Check sheet for the modelled part. Datum: model origin and axes. Units: mm. Face numbers are marked on the shaded views. A direction names the side the tool comes from. Round coordinates to 2 decimals unless told otherwise and drop trailing zeros.
Q1. Depth check by flat-ended pin: P1, Ø2, axis at x = 16, y = 59, coming from the +Z side; P2, Ø4, axis at x = 54.5, z = 3.5, coming from the -Y side; P3, Ø1.5, axis at x = 19.5, z = 23, coming from the -Y side. Enter the tip coordinate at first touch or a pass-through.
Q2. Set-up check for the marked faces 1 and 2: record each of +Z, -Z, +X, -X, +Y, -Y from which the full face is reachable in a straight line by a thin tool's end or side.
Q3. Scan lines: probe 1 along Y at (x, z) = (70.5, 4); probe 2 along Z at (x, y) = (26.5, 29); probe 3 along Z at (x, y) = (8.5, 72.5). Record each from-to range of solid material in increasing order.
Q4. Cross-section at A-A on x = 72.5. Give the number of separate pieces and of enclosed holes in the cut face, then the cut area to 3 significant figures.
Autodesk Fusion 360 part; units mm, degrees
sketch "Sketch1" plane through (0, 0, 0) normal (1, 0, 0) x (0, 1, 0)
  line L0 (0, 0) -> (90, 0)
  line L1 (0, 0) -> (77.7817, 77.7817)
  line L2 (77.7817, 77.7817) -> (81.3173, 74.2462)
  line L3 (81.3173, 74.2462) -> (12.0711, 5)
  line L4 (12.0711, 5) -> (90, 5)
  line L5 (90, 5) -> (90, 0)
  dimension "d1" = 110
  dimension "d2" = 5
  dimension "d3" = 5
  dimension "d4" = 45
  dimension "d5" = 90
extrude "Extrude1" add sketch "Sketch1" along normal blind 85
sketch "Sketch2" plane through (0, 0, 0) normal (0, -0.7071, 0.7071) x (1, 0, 0)
  line L0 (0, 110) -> (0, 0)
  line L1 (0, 0) -> (85, 0)
  line L2 (85, 0) -> (85, 110)
  line L3 (85, 110) -> (0, 110)
  line L4 (0, 12.0711) -> (85, 12.0711)
  line L5 (0, 0) -> (85, 0)
  line L6 (0, 17.0711) -> (85, 17.0711)
  line L7 (42.5, 17.0711) -> (42.5, 110) construction
  line L8 (42.5, 63.5355) -> (0, 63.5355) construction
  line L9 (15, 90) -> (70, 90)
  arc A0 (70, 90) -> (70, 100) centre (70, 95) ccw
  line L10 (70, 100) -> (15, 100)
  arc A1 (15, 100) -> (15, 90) centre (15, 95) ccw
  line L11 (15, 95) -> (70, 95) construction
  line L12 (70, 83.75) -> (15, 83.75)
  arc A2 (15, 83.75) -> (15, 73.75) centre (15, 78.75) ccw
  line L13 (15, 73.75) -> (70, 73.75)
  arc A3 (70, 73.75) -> (70, 83.75) centre (70, 78.75) ccw
  line L14 (70, 67.5) -> (15, 67.5)
  arc A4 (15, 67.5) -> (15, 57.5) centre (15, 62.5) ccw
  line L15 (15, 57.5) -> (70, 57.5)
  arc A5 (70, 57.5) -> (70, 67.5) centre (70, 62.5) ccw
  line L16 (70, 51.25) -> (15, 51.25)
  arc A6 (15, 51.25) -> (15, 41.25) centre (15, 46.25) ccw
  line L17 (15, 41.25) -> (70, 41.25)
  arc A7 (70, 41.25) -> (70, 51.25) centre (70, 46.25) ccw
  line L18 (70, 35) -> (15, 35)
  arc A8 (15, 35) -> (15, 25) centre (15, 30) ccw
  line L19 (15, 25) -> (70, 25)
  arc A9 (70, 25) -> (70, 35) centre (70, 30) ccw
  dimension "d8" = 5
  dimension "d51" = 10
  dimension "d52" = 10
  dimension "d53" = 10
  dimension "d54" = 5
  dimension "d57" = 0
  dimension "d58" = -65
extrude "Extrude2" add sketch "Sketch2" along normal blind 15 contours L0 L2 L4 L6
fillet "Fillet1" radius 2.5 1 edges at (42.5, 0, 0)
fillet "Fillet3" radius 5 1 edges at (42.5, 12.0711, 5)
fillet "Fillet4" radius 5 2 edges at (0, 79.5495, 76.014) (85, 79.5495, 76.014)
fillet "Fillet5" radius 5 2 edges at (85, -0.3033, 20.9099) (0, -0.3033, 20.9099)
sketch "Sketch3" plane through (0, 0, 5) normal (0, 0, 1) x (-1, 0, 0)
  line L0 (0, -24.1421) -> (-85, -24.1421)
  line L1 (-85, -24.1421) -> (-85, -90)
  line L2 (-85, -90) -> (0, -90)
  line L3 (0, -90) -> (0, -24.1421)
  line L4 (-42.5, -24.1421) -> (-42.5, -90) construction
  line L5 (-42.5, -57.0711) -> (-85, -57.0711) construction
  line L6 (-70, -44.1421) -> (-15, -44.1421)
  arc A0 (-15, -44.1421) -> (-15, -34.1421) centre (-15, -39.1421) ccw
  line L7 (-15, -34.1421) -> (-70, -34.1421)
  arc A1 (-70, -34.1421) -> (-70, -44.1421) centre (-70, -39.1421) ccw
  line L8 (-70, -39.1421) -> (-15, -39.1421) construction
  line L9 (-15, -54.1421) -> (-70, -54.1421)
  arc A2 (-70, -54.1421) -> (-70, -64.1421) centre (-70, -59.1421) ccw
  line L10 (-70, -64.1421) -> (-15, -64.1421)
  arc A3 (-15, -64.1421) -> (-15, -54.1421) centre (-15, -59.1421) ccw
  line L11 (-15, -74.1421) -> (-70, -74.1421)
  arc A4 (-70, -74.1421) -> (-70, -84.1421) centre (-70, -79.1421) ccw
  line L12 (-70, -84.1421) -> (-15, -84.1421)
  arc A5 (-15, -84.1421) -> (-15, -74.1421) centre (-15, -79.1421) ccw
  dimension "d61" = 10
  dimension "d62" = 10
  dimension "d63" = 10
  dimension "d64" = 5
  dimension "d67" = 0
  dimension "d68" = -40
fillet "Fillet6" radius 5 2 edges at (85, 90, 2.5) (0, 90, 2.5)
sketch "Sketch4" plane through (0, 8.5355, 8.5355) normal (0, -0.7071, -0.7071) x (1, 0, 0)
  arc A0 (5, 15) -> (0, 10) centre (5, 10) ccw
  line L0 (0, 10) -> (0, 0)
  line L1 (85, 0) -> (85, 10)
  arc A1 (85, 10) -> (80, 15) centre (80, 10) ccw
  line L2 (80, 15) -> (5, 15)
  line L3 (9, 4.5) -> (76, 4.5)
  arc A2 (76, 4.5) -> (76, 12.5) centre (76, 8.5) ccw
  line L4 (76, 12.5) -> (9, 12.5)
  arc A3 (9, 12.5) -> (9, 4.5) centre (9, 8.5) ccw
  line L5 (9, 8.5) -> (76, 8.5) construction
  line L6 (0, 0) -> (85, 0)
  dimension "d43" = 5
  dimension "d44" = 5
  dimension "d47" = 8
extrude "Extrude5" cut sketch "Sketch4" against normal up to surface (5 mm away) contours L3 A2 L4 A3
extrude "Extrude6" cut sketch "Sketch2" against normal up to surface (5 mm away) contours L9 A0 L10 A1 | L12 A2 L13 A3 | L14 A4 L15 A5 | L16 A6 L17 A7 | L18 A8 L19 A9
extrude "Extrude7" cut sketch "Sketch3" against normal up to surface (5 mm away) contours L6 A0 L7 A1 | L9 A2 L10 A3 | L11 A4 L12 A5
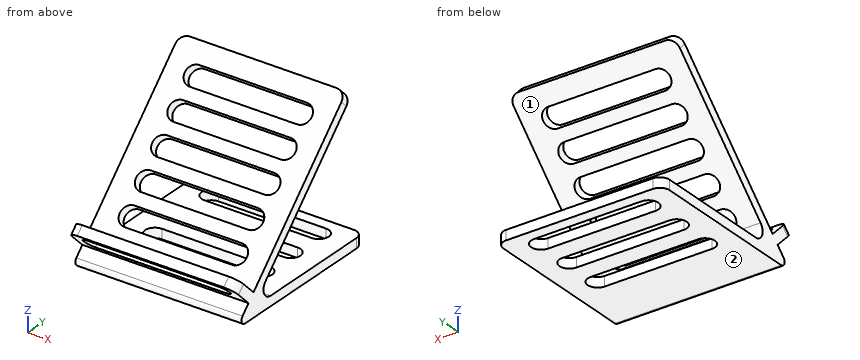
Results found:
1. P1: stops at z = 60
1. P2: stops at y = 3.54
1. P3: stops at y = 1.04
2. face 1: +X, -X, +Y
2. face 2: -Z, +X, -X, +Y, -Y
3. probe 1: y = 4.04 to 34.17, 44.12 to 54.17, 64.12 to 74.17, 84.12 to 90
3. probe 2: z = 0 to 5, 21.93 to 29
3. probe 3: z = 0 to 5, 65.43 to 72.5
4. separate pieces: 10
4. enclosed holes: 0
4. area: 651 mm2
